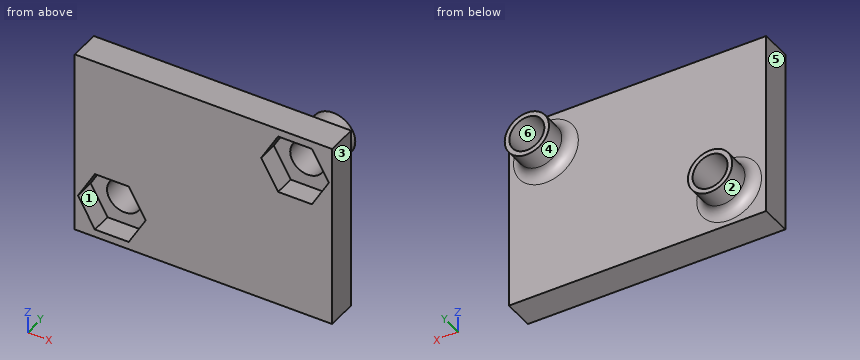
from build123d import *

# Parameters (mm, degrees)
SKETCH2_W           = 25
SKETCH2_H           = 18
BOSS_EXTRUDE1_DEPTH = 3
SKETCH3_R           = 1.7
CUT_EXTRUDE1_DEPTH  = 16.692354826
BOSS_EXTRUDE2_START = 3
SKETCH4_R           = 2.15
SKETCH4_R_2         = 1.7
BOSS_EXTRUDE2_DEPTH = 3
FILLET1_R           = 1
CUT_EXTRUDE2_DEPTH  = 2


with BuildPart() as part:
    # Sketch2 → Boss-Extrude1 (new body)
    with BuildSketch(Plane(origin=(0, 0, 0), x_dir=(1, 0, 0), z_dir=(0, 1, 0))):
        Rectangle(SKETCH2_W, SKETCH2_H)
    extrude(amount=BOSS_EXTRUDE1_DEPTH)

    # Sketch3 → Cut-Extrude1 (cut, through all)
    with BuildSketch(Plane(origin=(0, 3, 0), x_dir=(1, 0, 0), z_dir=(0, 1, 0))):
        with Locations(Location((-8.899893258, 5.4, 0), (0, 0, 270))):
            Circle(SKETCH3_R)
        with Locations(Location((8.899893258, -5.4, 0), (0, 0, 270))):
            Circle(SKETCH3_R)
    extrude(amount=-CUT_EXTRUDE1_DEPTH, mode=Mode.SUBTRACT)

    # Sketch4 → Boss-Extrude2 (add)
    # profile 1 of 2: a face of its own
    with BuildSketch(Plane(origin=(0, 3, 0), x_dir=(1, 0, 0), z_dir=(0, 1, 0)).offset(BOSS_EXTRUDE2_START)):
        with Locations(Location((-8.899893258, 5.4, 0), (0, 0, 270))):
            Circle(SKETCH4_R)
        with Locations(Location((-8.899893258, 5.4, 0), (0, 0, 270))):
            Circle(SKETCH4_R_2, mode=Mode.SUBTRACT)
    # profile 2 of 2: a face of its own
    with BuildSketch(Plane(origin=(0, 3, 0), x_dir=(1, 0, 0), z_dir=(0, 1, 0)).offset(BOSS_EXTRUDE2_START)):
        with Locations(Location((8.899893258, -5.4, 0), (0, 0, 270))):
            Circle(SKETCH4_R)
        with Locations(Location((8.899893258, -5.4, 0), (0, 0, 270))):
            Circle(SKETCH4_R_2, mode=Mode.SUBTRACT)
    extrude(amount=-BOSS_EXTRUDE2_DEPTH)

    # Fillet1
    fillet1_edges = [part.edges().sort_by_distance(p)[0] for p in [
        (-8.899893258, 3, -7.55),
        (8.899893258, 3, 3.25),
    ]]
    fillet(fillet1_edges, radius=FILLET1_R)

    # Sketch5 → Cut-Extrude2 (cut)
    with BuildSketch(Plane.XZ):
        Polygon((10.545341525, 2.55), (12.190789792, 5.4), (10.545341525, 8.25), (7.254444991, 8.25), (5.608996723, 5.4), (7.254444991, 2.55), align=None)
        Polygon((-7.254444991, -8.25), (-5.608996723, -5.4), (-7.254444991, -2.55), (-10.545341525, -2.55), (-12.190789792, -5.4), (-10.545341525, -8.25), align=None)
    extrude(amount=-CUT_EXTRUDE2_DEPTH, mode=Mode.SUBTRACT)


solid = part.part
Design review of the part built by this model. Coordinates are the model's own, in mm. Face numbers are marked on the shaded views. A direction names the side the tool comes from. Coordinates: 2 decimals unless noted, no trailing zeros. Loops run counter-clockwise (first coordinate to the right, second up) from the corner with the lowest first, then second, coordinate; pieces in that order, holes last. Notation, with made-up numbers: (50, 31) - (83, 31) arc R12 cw to (83, 51) - close; hole circle Ø2 at (-31, -21.5). An arc over 180 degrees is marked (long way). Use CSV: the item, a comma, the result in double quotes. Start each with the question number.
1. Add section D-D on x = 2.5. Give the boundary of the cut face in (y, z).
2. To check wall thickness, follow probe 1 along X at (y, z) = (4.35, -5.4); probe 2 along X at (y, z) = (2.85, 5.4); probe 3 along Y at (x, z) = (-2, -5). State the ranges of each line that lie inside material, in increasing order.
3. For the marked faces 1, 2 and 3, list the 3-axis set-ups (+Z, -Z, +X, -X, +Y, -Y) from which the entire face can be reached by the end or side of a thin tool; tool diameter is ignored.
4. Clearance check with a flat-ended pin moving along its axis: pin 1 (10 mm diameter, centred on x = 0.5, z = -2.5, fed in from +Y). State where the tip first meets the part, or that it passes through.
5. Mouldability with a two-part tool opening along Z and no side actions: class the marked faces 4, 5 and 6 as released by +Z, released by -Z, zero draft, split by the parting line, or undercut.
6. Add section C-C on z = -1. Give the boundary of the cut face in (x, y), plus the area to 3 significant figures.
7. Add section A-A on y = 0.85. Give the boundary of the cut face in (x, z), plus the area to 3 significant figures.
8. Add section B-B on y = 4.7. Give the boundary of the cut face in (x, z).
Resolved:
1,outline,"(0, -9) - (3, -9) - (3, 9) - (0, 9) - close"
2,probe 1,"-11.05 to -10.6, -7.2 to -6.75"
2,probe 2,"-12.5 to 7.2, 10.6 to 12.5"
2,probe 3,"0 to 3"
3,face 1,"-Y"
3,face 2,"+Y"
3,face 3,"+Z, -Z, +X, +Y, -Y"
4,pin 1,"y = 3"
5,face 4,"split by the parting line"
5,face 5,"zero draft"
5,face 6,"undercut"
6,outline,"(-12.5, 0) - (12.5, 0) - (12.5, 3) - (-12.5, 3) - close"
6,area,"75.0 mm2"
7,outline,"(-12.5, -9) - (12.5, -9) - (12.5, 9) - (-12.5, 9) - close; hole (-12.19, -5.4) - (-10.55, -8.25) - (-7.25, -8.25) - (-5.61, -5.4) - (-7.25, -2.55) - (-10.55, -2.55) - close; hole (5.61, 5.4) - (7.25, 2.55) - (10.55, 2.55) - (12.19, 5.4) - (10.55, 8.25) - (7.25, 8.25) - close"
7,area,"394 mm2"
8,outline,"circle Ø4.3 at (-8.9, -5.4); circle Ø4.3 at (8.9, 5.4); hole circle Ø3.4 at (-8.9, -5.4); hole circle Ø3.4 at (8.9, 5.4)"
